```python
from build123d import *

# Parameters (mm, degrees)
CUT_EXTRUDE1_DEPTH      = 73.886898686
CUT_EXTRUDE1_DEPTH_BACK = 73.886898686
SKETCH2_R               = 38.1
CUT_EXTRUDE2_DEPTH      = 73.886898754
CUT_EXTRUDE2_DEPTH_BACK = 73.886898754
SKETCH3_R               = 4.7625
SKETCH7_R               = 4.7625
CUT_EXTRUDE5_DEPTH      = 22.5
CUT_EXTRUDE3_DEPTH      = 73.886898857
CUT_EXTRUDE3_DEPTH_BACK = 73.886898857
SKETCH4_R               = 3.175
SKETCH4_R_2             = 2.58
SKETCH5_R               = 16.94
CUT_EXTRUDE4_DEPTH      = 63.461988614
SKETCH8_R               = 2.5
CUT_EXTRUDE6_DEPTH      = 20
SKETCH9_R               = 9
CUT_EXTRUDE7_DEPTH      = 18


with BuildPart() as part:
    # Sketch1 → Revolve1 (revolve)
    with BuildSketch(Plane.XY, mode=Mode.PRIVATE) as revolve1_sk:
        Polygon((0, 0), (37.5, 0), (37.5, 33), (30, 33), (30, 50), (0, 50), align=None)
    revolve(revolve1_sk.sketch.rotate(Axis((0, 50, 0), (0, -1, 0)), 180), axis=Axis((0, 50, 0), (0, -1, 0)))

    # Sketch2 → Cut-Extrude1 (cut, two sides: drawn at the far end of the back side and taken through both)
    with BuildSketch(Plane.XY.offset(-CUT_EXTRUDE1_DEPTH_BACK)):
        with Locations((0, 73.486379031)):
            Circle(SKETCH2_R)
    extrude(amount=CUT_EXTRUDE1_DEPTH + CUT_EXTRUDE1_DEPTH_BACK, mode=Mode.SUBTRACT)

    # Sketch3 → Cut-Extrude2 (cut, two sides: drawn at the far end of the back side and taken through both)
    with BuildSketch(Plane.XZ.offset(-CUT_EXTRUDE2_DEPTH_BACK)):
        Circle(SKETCH3_R)
    extrude(amount=CUT_EXTRUDE2_DEPTH + CUT_EXTRUDE2_DEPTH_BACK, mode=Mode.SUBTRACT)

    # Sketch7 → Cut-Extrude5 (cut)
    with BuildSketch(Plane(origin=(-26.516504294, 0, 26.516504294), x_dir=(0, 1, 0), z_dir=(-0.7071067811865464, 0, 0.7071067811865488))):
        with Locations(Location((16.5, 0, 0), (0, 0, 270))):
            Circle(SKETCH7_R)
    extrude(amount=-CUT_EXTRUDE5_DEPTH, mode=Mode.SUBTRACT)

    # Sketch4 → Cut-Extrude3 (cut, two sides: drawn at the far end of the back side and taken through both)
    with BuildSketch(Plane.XZ.offset(-CUT_EXTRUDE3_DEPTH_BACK)):
        with Locations((0, 23.825)):
            Circle(SKETCH4_R)
        with Locations((0, -23.825)):
            Circle(SKETCH4_R)
        with Locations((-14.225, 0)):
            Circle(SKETCH4_R_2)
        with Locations((0, 14.225)):
            Circle(SKETCH4_R_2)
        with Locations((14.225, 0)):
            Circle(SKETCH4_R_2)
        with Locations((0, -14.225)):
            Circle(SKETCH4_R_2)
    extrude(amount=CUT_EXTRUDE3_DEPTH + CUT_EXTRUDE3_DEPTH_BACK, mode=Mode.SUBTRACT)

    # Sketch5 → Cut-Extrude4 (cut, through all)
    with BuildSketch(Plane(origin=(0, 33, 0), x_dir=(1, 0, 0), z_dir=(0, 1, 0))):
        Circle(SKETCH5_R)
    extrude(amount=CUT_EXTRUDE4_DEPTH, mode=Mode.SUBTRACT)

    # Sketch8 → Cut-Extrude6 (cut)
    with BuildSketch(Plane(origin=(0, 33, 0), x_dir=(1, 0, 0), z_dir=(0, 1, 0))):
        with Locations(Location((-10.058593962, -10.058593962, 0), (0, 0, 180))):
            Circle(SKETCH8_R)
    extrude(amount=-CUT_EXTRUDE6_DEPTH, mode=Mode.SUBTRACT)

    # Sketch9 → Cut-Extrude7 (cut)
    with BuildSketch(Plane.XZ):
        Circle(SKETCH9_R)
    extrude(amount=-CUT_EXTRUDE7_DEPTH, mode=Mode.SUBTRACT)


solid = part.part
```
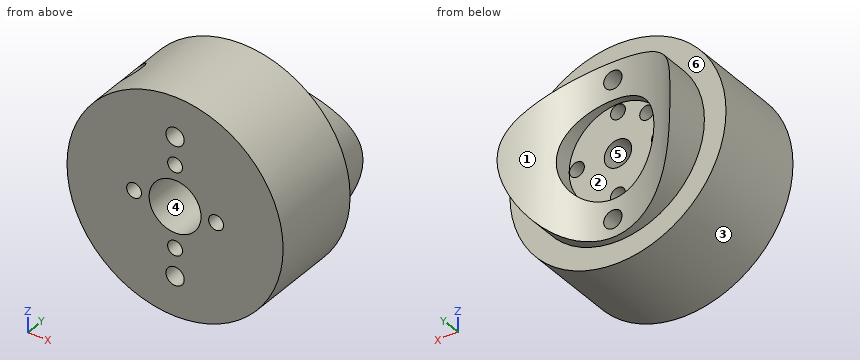
For this review, take the finished solid that the model builds, in its own axes (mm). Face numbers are marked on the shaded views. A direction names the side the tool comes from. Round coordinates to 2 decimals unless told otherwise and drop trailing zeros. Write each loop counter-clockwise with the first axis right and the second up, starting at its lowest first coordinate (ties: lowest second). Pieces come first, ordered by that corner, then holes. Notation, with made-up numbers: (75, 37) - (124, 37) arc R15 cw to (124, 54) - close; hole circle Ø4 at (16, 78.25). An arc over 180 degrees is marked (long way). Answer as a JSON object with one key per item and string values.
1. Draft analysis for pull direction Z (two halves, no side actions). For the marked faces 3, 4, 5 and 6, state which applies: +Z half, -Z half, draft (parallel to the pull), parting line (faces both ways), or undercut.
Response values:
{"face 3": "parting line", "face 4": "undercut", "face 5": "undercut", "face 6": "draft"}
2. We need section B-B on z = -13. Give the boundary of the cut face in (x, y), then the cut area to 3 significant figures.
Response values:
{"outline": "(-35.17, 0) - (-2.27, 0) - (-2.27, 33) - (-10.86, 33) - (-10.86, 36.97) arc R38.1 cw to (-27.04, 46.64) - (-27.04, 33) - (-35.17, 33) - close; (2.27, 0) - (35.17, 0) - (35.17, 33) - (27.04, 33) - (27.04, 46.64) arc R38.1 cw to (10.86, 36.97) - (10.86, 33) - (2.27, 33) - close", "area": "2,430 mm2"}
3. We need section D-D on y = 8. Give the boundary of the cut face in (x, z) (3 decimals), then the cut area to 3 significant figures.
Response values:
{"outline": "circle Ø75 at (0, 0); hole circle Ø5.16 at (-14.225, 0); hole circle Ø18 at (0, 0); hole circle Ø6.35 at (0, -23.825); hole circle Ø6.35 at (0, 23.825); hole circle Ø5.16 at (0, -14.225); hole circle Ø5.16 at (0, 14.225); hole circle Ø5.16 at (14.225, 0)", "area": "4,020 mm2"}
4. We need section A-A on z = 0. Count the separate pieces of the cut face and the enclosed holes in it, then the cut area to 3 significant figures.
Response values:
{"separate pieces": "4", "enclosed holes": "0", "area": "1,950 mm2"}
5. To check wall thickness, follow line 1 along Z through (x, y) = (0, 34); line 2 along X through (y, z) = (32.5, 0.5); line 3 along X through (y, z) = (12, -0.5). State the ranges of each line that lie inside material, in increasing order.
Response values:
{"line 1": "z = -30 to -27, -20.65 to -16.94, 16.94 to 20.65, 27 to 30", "line 2": "x = -37.5 to -16.76, -11.69 to -4.74, 4.74 to 11.69, 16.76 to 37.5", "line 3": "x = -37.5 to -16.76, -11.69 to -8.99, 8.99 to 11.69, 16.76 to 37.5"}
6. Tool access review of the marked faces 1 and 2: name each direction out of +Z, -Z, +X, -X, +Y, -Y from which nothing blocks a thin tool from reaching the whole face with its end or side.
Response values:
{"face 1": "+Z, -Z, +Y", "face 2": "+Y"}
7. For pin 1 Ø6 at (x, z) = (0, 14.225) entering from +Y; pin 2 Ø10 at (y, z) = (24.5, 10) entering from +X; pin 3 Ø6 at (x, z) = (-18, 10) entering from +Y; pin 4 Ø4 at (x, z) = (0, -23.825) entering from -Y, all flat-tipped, find the tip position at first contact; note any pin that passes through.
Response values:
{"pin 1": "stops at y = 35.41", "pin 2": "stops at x = 37.17", "pin 3": "stops at y = 41.7", "pin 4": "passes through"}
